Read the model definition and answer for the solid it produces. Units are mm, in the model's axes. Give positions to 0.01 mm unless a question says otherwise; leave off trailing zeros. Write each loop counter-clockwise with the first axis right and the second up, starting at its lowest first coordinate (ties: lowest second). Pieces come first, ordered by that corner, then holes. Notation, with made-up numbers: M 38,-35 L 77,-35 A16 ccw 77,-14 Z; hole C -22,59 d4. An arc over 180 degrees is marked long. Use a Markdown table: item, result. Add a question column.
Item 1: A cutting plane is placed at A-A on y = -17.5. Determine the outline of the cut face in (x, z).
Item 2: A cutting plane is placed at C-C on y = -5.5. Determine the outline of the cut face in (x, z).
Item 3: A cutting plane is placed at B-B on x = 86.5. Determine the outline of the cut face in (y, z), then the cut area to 3 significant figures.
Item 4: A cutting plane is placed at D-D on x = -44.5. Determine the outline of the cut face in (y, z), then the cut area to 3 significant figures.
Item 5: Consider probe 1 along Z at (x, y) = (52, -30.5); probe 2 along X at (y, z) = (15.5, 12.5); probe 3 along X at (y, z) = (-16, 15.5). Determine where each line is inside the solid, lowest interval first. Write a range as [from, to].
Item 6: Given P1, Ø4, axis at x = 0.5, y = -26, coming from the -Z side; P2, Ø4.5, axis at x = 96, y = 17.5, coming from the +Z side; P3, Ø4.5, axis at x = 0, y = -25, coming from the -Z side; P4, Ø1.5, axis at x = -18.5, z = 7, coming from the -Y side, each flat-ended and moving along its own axis, determine where each tip first touches the part or whether it passes through.
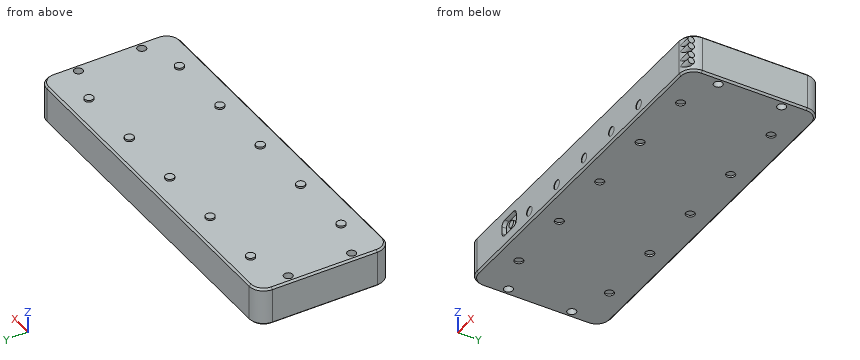
from build123d import *

# Parameters (mm, degrees)
SKETCH1_W           = 201
SKETCH1_H           = 74
BOSS_EXTRUDE1_DEPTH = 21
FILLET1_R           = 8
CHAMFER1_SIZE       = 1
CUT_EXTRUDE1_REACH  = 111.134
SKETCH2_R           = 2.4
SKETCH3_R           = 2.4
BOSS_EXTRUDE2_DEPTH = 1
BOSS_EXTRUDE6_REACH = 207.558
SKETCH4_R           = 1.75
SKETCH5_R           = 2.4
CUT_EXTRUDE2_DEPTH  = 1
SKETCH6_W           = 13
SKETCH6_H           = 9
CUT_EXTRUDE3_DEPTH  = 2.4
SKETCH7_R           = 2
BOSS_EXTRUDE7_DEPTH = 1.25
FILLET2_R           = 2.5
SKETCH8_R           = 2.5
CUT_EXTRUDE4_DEPTH  = 0.25
LPATTERN1_COUNT     = 5
LPATTERN1_PITCH     = 25


with BuildPart() as part:
    # Sketch1 → Boss-Extrude1 (new body)
    with BuildSketch(Plane.XY):
        Rectangle(SKETCH1_W, SKETCH1_H)
    extrude(amount=BOSS_EXTRUDE1_DEPTH)

    # Fillet1
    fillet1_edges = [part.edges().sort_by_distance(p)[0] for p in [
        (100.5, -37, 10.5),
        (-100.5, -37, 10.5),
        (-100.5, 37, 10.5),
        (100.5, 37, 10.5),
    ]]
    fillet(fillet1_edges, radius=FILLET1_R)

    # Chamfer1
    chamfer1_edges = [part.edges().sort_by_distance(p)[0] for p in [
        (0, 37, 0),
        (0, 37, 21),
        (100.5, 0, 0),
        (0, -37, 0),
        (-100.5, 0, 0),
        (-98.156854249, 34.656854249, 0),
        (-98.156854249, -34.656854249, 0),
        (98.156854249, -34.656854249, 0),
        (98.156854249, 34.656854249, 0),
        (100.5, 0, 21),
        (-100.5, 0, 21),
        (0, -37, 21),
        (-98.156854249, 34.656854249, 21),
        (-98.156854249, -34.656854249, 21),
        (98.156854249, -34.656854249, 21),
        (98.156854249, 34.656854249, 21),
    ]]
    chamfer(chamfer1_edges, length=CHAMFER1_SIZE)

    # Sketch2 → Cut-Extrude1 (cut, up to next)
    with BuildSketch(Plane.XY.offset(21), mode=Mode.PRIVATE) as cut_extrude1_sk1:
        with Locations((-96, 17.5)):
            Circle(SKETCH2_R)
    cut_extrude1_tool1 = extrude(cut_extrude1_sk1.sketch, amount=-CUT_EXTRUDE1_REACH, mode=Mode.PRIVATE) & part.part
    # Sketch2 → Cut-Extrude1 (cut, up to next)
    with BuildSketch(Plane.XY.offset(21), mode=Mode.PRIVATE) as cut_extrude1_sk2:
        with Locations((-96, -17.5)):
            Circle(SKETCH2_R)
    cut_extrude1_tool2 = extrude(cut_extrude1_sk2.sketch, amount=-CUT_EXTRUDE1_REACH, mode=Mode.PRIVATE) & part.part
    # Sketch2 → Cut-Extrude1 (cut, up to next)
    with BuildSketch(Plane.XY.offset(21), mode=Mode.PRIVATE) as cut_extrude1_sk3:
        with Locations(Location((96, 17.5, 0), (0, 0, 180))):
            Circle(SKETCH2_R)
    cut_extrude1_tool3 = extrude(cut_extrude1_sk3.sketch, amount=-CUT_EXTRUDE1_REACH, mode=Mode.PRIVATE) & part.part
    # Sketch2 → Cut-Extrude1 (cut, up to next)
    with BuildSketch(Plane.XY.offset(21), mode=Mode.PRIVATE) as cut_extrude1_sk4:
        with Locations(Location((96, -17.5, 0), (0, 0, 180))):
            Circle(SKETCH2_R)
    cut_extrude1_tool4 = extrude(cut_extrude1_sk4.sketch, amount=-CUT_EXTRUDE1_REACH, mode=Mode.PRIVATE) & part.part
    add(cut_extrude1_tool1.solids().sort_by_distance((-96, 17.5, 21))[0], mode=Mode.SUBTRACT)
    add(cut_extrude1_tool2.solids().sort_by_distance((-96, -17.5, 21))[0], mode=Mode.SUBTRACT)
    add(cut_extrude1_tool3.solids().sort_by_distance((96, 17.5, 21))[0], mode=Mode.SUBTRACT)
    add(cut_extrude1_tool4.solids().sort_by_distance((96, -17.5, 21))[0], mode=Mode.SUBTRACT)

    # Sketch3 → Boss-Extrude2 (add)
    with BuildSketch(Plane.XY.offset(21)):
        with Locations(Location((0, 25, 0), (0, 0, 180))):
            Circle(SKETCH3_R)
        with Locations(Location((0, -25, 0), (0, 0, 180))):
            Circle(SKETCH3_R)
        with Locations(Location((-74, 25, 0), (0, 0, 180))):
            Circle(SKETCH3_R)
        with Locations(Location((-37, 25, 0), (0, 0, 180))):
            Circle(SKETCH3_R)
        with Locations(Location((37, 25, 0), (0, 0, 180))):
            Circle(SKETCH3_R)
        with Locations(Location((74, 25, 0), (0, 0, 180))):
            Circle(SKETCH3_R)
        with Locations(Location((74, -25, 0), (0, 0, 180))):
            Circle(SKETCH3_R)
        with Locations(Location((37, -25, 0), (0, 0, 180))):
            Circle(SKETCH3_R)
        with Locations(Location((-37, -25, 0), (0, 0, 180))):
            Circle(SKETCH3_R)
        with Locations(Location((-74, -25, 0), (0, 0, 180))):
            Circle(SKETCH3_R)
    extrude(amount=BOSS_EXTRUDE2_DEPTH)

    # Sketch4 → Boss-Extrude6 (add, up to next)
    with BuildSketch(Plane(origin=(100.5, 0, 0), x_dir=(0, 0, -1), z_dir=(1, 0, 0)), mode=Mode.PRIVATE) as boss_extrude6_sk1:
        with Locations((-16.6, -35.15)):
            Circle(SKETCH4_R)
    boss_extrude6_tool1 = extrude(boss_extrude6_sk1.sketch, amount=-BOSS_EXTRUDE6_REACH, mode=Mode.PRIVATE) - part.part
    # Sketch4 → Boss-Extrude6 (add, up to next)
    with BuildSketch(Plane(origin=(100.5, 0, 0), x_dir=(0, 0, -1), z_dir=(1, 0, 0)), mode=Mode.PRIVATE) as boss_extrude6_sk2:
        with Locations((-13, -35.15)):
            Circle(SKETCH4_R)
    boss_extrude6_tool2 = extrude(boss_extrude6_sk2.sketch, amount=-BOSS_EXTRUDE6_REACH, mode=Mode.PRIVATE) - part.part
    # Sketch4 → Boss-Extrude6 (add, up to next)
    with BuildSketch(Plane(origin=(100.5, 0, 0), x_dir=(0, 0, -1), z_dir=(1, 0, 0)), mode=Mode.PRIVATE) as boss_extrude6_sk3:
        with Locations((-8, -35.15)):
            Circle(SKETCH4_R)
    boss_extrude6_tool3 = extrude(boss_extrude6_sk3.sketch, amount=-BOSS_EXTRUDE6_REACH, mode=Mode.PRIVATE) - part.part
    # Sketch4 → Boss-Extrude6 (add, up to next)
    with BuildSketch(Plane(origin=(100.5, 0, 0), x_dir=(0, 0, -1), z_dir=(1, 0, 0)), mode=Mode.PRIVATE) as boss_extrude6_sk4:
        with Locations((-4.4, -35.15)):
            Circle(SKETCH4_R)
    boss_extrude6_tool4 = extrude(boss_extrude6_sk4.sketch, amount=-BOSS_EXTRUDE6_REACH, mode=Mode.PRIVATE) - part.part
    add(boss_extrude6_tool1.solids().sort_by_distance((100.5, -35.15, 16.6))[0])
    add(boss_extrude6_tool2.solids().sort_by_distance((100.5, -35.15, 13))[0])
    add(boss_extrude6_tool3.solids().sort_by_distance((100.5, -35.15, 8))[0])
    add(boss_extrude6_tool4.solids().sort_by_distance((100.5, -35.15, 4.4))[0])

    # Sketch5 → Cut-Extrude2 (cut)
    with BuildSketch(Plane(origin=(0, 0, 0), x_dir=(-1, 0, 0), z_dir=(0, 0, -1))):
        with Locations((0, 25)):
            Circle(SKETCH5_R)
        with Locations((0, -25)):
            Circle(SKETCH5_R)
        with Locations((-74, 25)):
            Circle(SKETCH5_R)
        with Locations((-37, 25)):
            Circle(SKETCH5_R)
        with Locations((37, 25)):
            Circle(SKETCH5_R)
        with Locations((74, 25)):
            Circle(SKETCH5_R)
        with Locations((74, -25)):
            Circle(SKETCH5_R)
        with Locations((37, -25)):
            Circle(SKETCH5_R)
        with Locations((-37, -25)):
            Circle(SKETCH5_R)
        with Locations((-74, -25)):
            Circle(SKETCH5_R)
    extrude(amount=-CUT_EXTRUDE2_DEPTH, mode=Mode.SUBTRACT)

    # Sketch6 → Cut-Extrude3 (cut)
    with BuildSketch(Plane.XZ.offset(37)):
        with Locations((-63, 10.5)):
            Rectangle(SKETCH6_W, SKETCH6_H)
    extrude(amount=-CUT_EXTRUDE3_DEPTH, mode=Mode.SUBTRACT)

    # Sketch7 → Boss-Extrude7 (add)
    with BuildSketch(Plane.XZ.offset(34.6)):
        with Locations(Location((-63, 10.5, 0), (0, 0, 270))):
            Circle(SKETCH7_R)
    extrude(amount=BOSS_EXTRUDE7_DEPTH)

    # Fillet2
    fillet2_edges = [part.edges().sort_by_distance(p)[0] for p in [
        (-56.5, -35.8, 15),
        (-56.5, -35.8, 6),
        (-69.5, -35.8, 6),
        (-69.5, -35.8, 15),
    ]]
    fillet(fillet2_edges, radius=FILLET2_R)

    # Sketch8 → Cut-Extrude4 (cut)
    with BuildSketch(Plane.XZ.offset(37)):
        with Locations(Location((55.5, 6, 0), (0, 0, 270))):
            Circle(SKETCH8_R)
    cut_extrude4 = extrude(amount=-CUT_EXTRUDE4_DEPTH, mode=Mode.SUBTRACT)

    # LPattern1: Cut-Extrude4 ×5
    with Locations(*[(-i * LPATTERN1_PITCH, 0, 0) for i in range(1, LPATTERN1_COUNT)]):
        add(cut_extrude4, mode=Mode.SUBTRACT)


solid = part.part
Filled in:
| question | item | result |
|---|---|---|
| 1 | outline | M -100.5,1 L -99.5,0 L -98.4,0 L -98.4,21 L -99.5,21 L -100.5,20 Z; M -93.6,0 L 93.6,0 L 93.6,21 L -93.6,21 Z; M 98.4,0 L 99.5,0 L 100.5,1 L 100.5,20 L 99.5,21 L 98.4,21 Z |
| 2 | outline | M -100.5,1 L -99.5,0 L 99.5,0 L 100.5,1 L 100.5,20 L 99.5,21 L -99.5,21 L -100.5,20 Z |
| 3 | outline | M -37,1 L -36,0 L 36,0 L 37,1 L 37,20 L 36,21 L -36,21 L -37,20 Z |
| 3 | area | 1,550 mm² |
| 4 | outline | M -37,1 L -36,0 L 36,0 L 37,1 L 37,20 L 36,21 L -36,21 L -37,20 L -37,8.5 L -36.75,8.5 L -36.75,3.5 L -37,3.5 Z |
| 4 | area | 1,550 mm² |
| 5 | probe 1 | [0, 21] |
| 5 | probe 2 | [-100.5, -97.33], [-94.67, 94.67], [97.33, 100.5] |
| 5 | probe 3 | [-100.5, -97.87], [-94.13, 94.13], [97.87, 100.5] |
| 6 | P1 | z = 0 |
| 6 | P2 | through |
| 6 | P3 | z = 1 |
| 6 | P4 | y = -36.75 |
